from build123d import *

# Parameters (mm, degrees)
F0_R     = 83.5
F1_DEPTH = 20


with BuildPart() as f1:
    # F0 (on Front) → F1 (new body)
    with BuildSketch(Plane.XZ):
        with BuildLine():
            ThreePointArc((-31.60529, -85.868246), (-25.730746, -99.97979), (-11.605346, -105.820939))
            Line((-11.605346, -105.820939), (11.605346, -105.820939))
            ThreePointArc((11.605346, -105.820939), (25.730746, -99.97979), (31.60529, -85.868246))
            ThreePointArc((31.60529, -85.868246), (91.499987, -0.048384), (31.696085, 85.834773))
            Line((31.696085, 85.834773), (32.388896, 105.820939))
            Line((32.388896, 105.820939), (21.988716, 105.820939))
            Line((21.988716, 105.820939), (21.988716, 116.298988))
            Line((21.988716, 116.298988), (-60.078114, 116.298988))
            Line((-60.078114, 116.298988), (-60.078114, 95.342889))
            Line((-60.078114, 95.342889), (-31.696085, 95.342889))
            Line((-31.696085, 95.342889), (-31.696085, 85.834773))
            ThreePointArc((-31.696085, 85.834773), (-91.499987, -0.048384), (-31.60529, -85.868246))
        make_face()
        Circle(F0_R, mode=Mode.SUBTRACT)
    extrude(amount=F1_DEPTH)


solid = f1.part
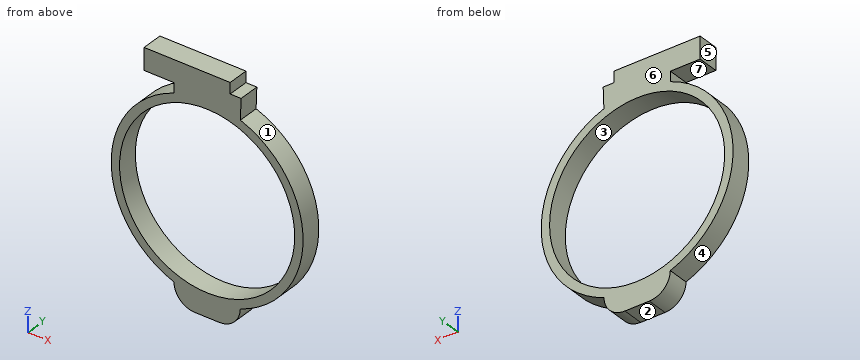
Geometry check sheet. Reference: the model listing, model coordinates, mm. Face numbers are marked on the shaded views. A direction names the side the tool comes from. Round coordinates to 2 decimals unless told otherwise and drop trailing zeros. Loops run counter-clockwise (first coordinate to the right, second up) from the corner with the lowest first, then second, coordinate; pieces in that order, holes last. Notation, with made-up numbers: (76, 38.25) - (86, 38.25) arc R26 ccw to (86, 58.25) - close; hole circle Ø7 at (35.25, 51.5). An arc over 180 degrees is marked (long way). One line per question, with ' | ' between items. Start each with the question number.
1. Tool access check on the marked faces 5, 6 and 7. Record the directions out of +Z, -Z, +X, -X, +Y, -Y that give a thin tool (end or side, any length) a straight path to the whole face; none if there is none.
2. Cross-section at C-C on y = -14.5. Record the cut outline in (x, z), then the cut area to 3 significant figures.
3. Scan lines: line 1 (Z direction, x = -2.5, y = -12.75); line 2 (Z direction, x = -36, y = -17.5); line 3 (X direction, y = -6.25, z = 54). Record each from-to range of solid material in increasing order. Write a range as [from, to].
4. Cross-section at D-D on x = -50. Record the cut outline in (y, z).
5. Depth check by flat-ended pin: pin 1 (3 mm diameter, centred on x = 72, y = -15, fed in from -Z); pin 2 (10 mm diameter, centred on x = 22.5, y = -3.5, fed in from -Z); pin 3 (5 mm diameter, centred on y = -9, z = 91.5, fed in from -X). Enter the tip coordinate at first touch or a pass-through.
6. Draft check along X on the marked faces 1, 2, 3 and 4. Enter one of: released by +X, released by -X, zero draft, split by the parting line, or undercut.
7. Cross-section at B-B on z = 0. Record the cut outline in (x, y), then the cut area to 3 significant figures.
8. Cross-section at A-A on x = 0. Record the cut outline in (y, z).
Taken from the geometry:
1) face 5: +Z, -X, +Y, -Y | face 6: +Z, -Z, +X, -X, +Y | face 7: -X, +Y, -Y
2) outline: (-60.08, 95.34) - (-31.7, 95.34) - (-31.7, 85.83) arc R91.5 ccw to (-31.61, -85.87) arc R20 ccw to (-11.61, -105.82) - (11.61, -105.82) arc R20 ccw to (31.61, -85.87) arc R91.5 ccw to (31.7, 85.83) - (32.39, 105.82) - (21.99, 105.82) - (21.99, 116.3) - (-60.08, 116.3) - close; hole circle Ø167 at (0, 0) | area: 7,440 mm²
3) line 1: [-105.82, -83.46], [83.46, 116.3] | line 2: [-84.12, -75.34], [75.34, 84.12], [95.34, 116.3] | line 3: [-73.87, -63.69], [63.69, 73.87]
4) outline: (-20, -76.63) - (0, -76.63) - (0, -66.87) - (-20, -66.87) - close; (-20, 66.87) - (0, 66.87) - (0, 76.63) - (-20, 76.63) - close; (-20, 95.34) - (0, 95.34) - (0, 116.3) - (-20, 116.3) - close
5) pin 1: z = -58.33 | pin 2: z = -104.93 | pin 3: x = -31.7
6) face 1: released by +X | face 2: zero draft | face 3: undercut | face 4: released by -X
7) outline: (-91.5, -20) - (-83.5, -20) - (-83.5, 0) - (-91.5, 0) - close; (83.5, -20) - (91.5, -20) - (91.5, 0) - (83.5, 0) - close | area: 320 mm²
8) outline: (-20, -105.82) - (0, -105.82) - (0, -83.5) - (-20, -83.5) - close; (-20, 83.5) - (0, 83.5) - (0, 116.3) - (-20, 116.3) - close
